Read the model definition and answer for the solid it produces. Units are mm, in the model's axes. A direction names the side the tool comes from. Coordinates: 2 decimals unless noted, no trailing zeros. Write each loop counter-clockwise with the first axis right and the second up, starting at its lowest first coordinate (ties: lowest second). Pieces come first, ordered by that corner, then holes.
(1) Which of the six approach directions +Z, -Z, +X, -X, +Y, -Y give full straight-line access (tool end or side, diameter ignored) to faces 4 (the flat face through (-0.58, 10, -10.35)), 5 (the flat face through (-0.55, 0, -10.35)), 6 (the flat face through (0, 5, -10.2))?
(2) The part is cut by section A-A, the plane x = -24.5. Determine the outline of the cut face in (y, z), and give its area (3 significant figures).
(3) The part is cut by section C-C, the plane z = -5. State how many separate pieces and enclosed holes the cut face has, and give its area (3 significant figures).
(4) The part is cut by section B-B, the plane y = 2.75. Determine the outline of the cut face in (x, z).
(5) Straight lines are drawn through the part: line 1 along X through (y, z) = (4, 5); line 2 along X through (y, z) = (-6.5, -9); line 3 along X through (y, z) = (2.5, 7). For each, find the intervals that lie inside material, in ascending order.
(6) Determine the mould class of faces 1 (the cylindrical face through (-43, -9, 5.8)), 2 (the cylindrical face through (-45.07, -2.68, -13.7)), 3 (the cylindrical face through (-45.07, 8.5, -0.21)) for opening direction Z: pulls with the +Z half, pulls with the -Z half, needs draft (parallel to the pull), parting line crosses it, or undercut.
(7) Given pin 1 (15 mm diameter, centred on x = -16, z = -4, fed in from -Y); pin 2 (1.5 mm diameter, centred on y = 7, z = 3.5, fed in from -X), each flat-ended and moving along its own axis, determine where each tip first touches the part or whether it passes through.
(8) The part is cut by section D-D, the plane y = -2.5. Determine the outline of the cut face in (x, z).
```python
from build123d import *

# Parameters (mm, degrees)
SKETCH_1_W          = 93
SKETCH_1_H          = 30.4
SKETCH_1_R          = 2.2
SKETCH_1_W_2        = 40.4
SKETCH_1_H_2        = 20.4
EXTRUDE_1_DEPTH     = 10
SKETCH_2_W          = 7
SKETCH_2_H          = 30.4
EXTRUDE_2_DEPTH     = 15
SKETCH_4_R          = 1.7
CUT_EXTRUDE_2_DEPTH = 96.420333263
FILLET_1_R          = 5


with BuildPart() as part:
    # 草图1 → 凸台-拉伸1 (new body)
    with BuildSketch(Plane(origin=(0, 0, 0), x_dir=(1, 0, 0), z_dir=(0, 1, 0))):
        Rectangle(SKETCH_1_W, SKETCH_1_H)
        with Locations(Location((-24.5, 5, 0), (0, 0, 270))):
            Circle(SKETCH_1_R, mode=Mode.SUBTRACT)
        with Locations(Location((-24.5, -5, 0), (0, 0, 270))):
            Circle(SKETCH_1_R, mode=Mode.SUBTRACT)
        with Locations(Location((24.5, -5, 0), (0, 0, 270))):
            Circle(SKETCH_1_R, mode=Mode.SUBTRACT)
        with Locations(Location((24.5, 5, 0), (0, 0, 270))):
            Circle(SKETCH_1_R, mode=Mode.SUBTRACT)
        Rectangle(SKETCH_1_W_2, SKETCH_1_H_2, mode=Mode.SUBTRACT)
    extrude(amount=EXTRUDE_1_DEPTH)

    # 草图2 → 凸台-拉伸2 (add)
    with BuildSketch(Plane.XZ):
        with Locations((-43, 0)):
            Rectangle(SKETCH_2_W, SKETCH_2_H)
        with Locations((43, 0)):
            Rectangle(SKETCH_2_W, SKETCH_2_H)
    extrude(amount=EXTRUDE_2_DEPTH)

    # 草图4 → 切除-拉伸2 (cut, through all)
    with BuildSketch(Plane.ZY.offset(46.5)):
        with Locations((-5, -7.5)):
            Circle(SKETCH_4_R)
        with Locations((5, -7.5)):
            Circle(SKETCH_4_R)
    extrude(amount=-CUT_EXTRUDE_2_DEPTH, mode=Mode.SUBTRACT)

    # 圆角1
    fillet_1_edges = [part.edges().sort_by_distance(p)[0] for p in [
        (46.5, 10, 0),
        (-46.5, 10, 0),
        (-46.5, -2.5, -15.2),
        (46.5, -2.5, -15.2),
        (46.5, -2.5, 15.2),
        (-46.5, -2.5, 15.2),
    ]]
    fillet(fillet_1_edges, radius=FILLET_1_R)


solid = part.part
```
Computed:
1. face 4: +Z, -Z, +X, -X, +Y
1. face 5: +Z, -Z, -Y
1. face 6: +Y, -Y
2. outline: (0, -15.2) - (10, -15.2) - (10, -7.2) - (0, -7.2) - close; (0, -2.8) - (10, -2.8) - (10, 2.8) - (0, 2.8) - close; (0, 7.2) - (10, 7.2) - (10, 15.2) - (0, 15.2) - close
2. area: 216 mm2
3. separate pieces: 6
3. enclosed holes: 0
3. area: 590 mm2
4. outline: (-46.5, -10.2) arc R5 ccw to (-41.5, -15.2) - (41.5, -15.2) arc R5 ccw to (46.5, -10.2) - (46.5, 10.2) arc R5 ccw to (41.5, 15.2) - (-41.5, 15.2) arc R5 ccw to (-46.5, 10.2) - close; hole circle Ø4.4 at (-24.5, -5); hole circle Ø4.4 at (-24.5, 5); hole (-20.2, -10.2) - (20.2, -10.2) - (20.2, 10.2) - (-20.2, 10.2) - close; hole circle Ø4.4 at (24.5, -5); hole circle Ø4.4 at (24.5, 5)
5. line 1: x = -46.5 to -26.7, -22.3 to -20.2, 20.2 to 22.3, 26.7 to 46.5
5. line 2: x = -46.5 to -39.5, 39.5 to 46.5
5. line 3: x = -46.5 to -25.42, -23.58 to -20.2, 20.2 to 23.58, 25.42 to 46.5
6. face 1: undercut
6. face 2: pulls with the -Z half
6. face 3: needs draft
7. pin 1: stops at y = 0
7. pin 2: stops at x = -46.34
8. outline: (-46.5, -10.2) arc R5 ccw to (-41.5, -15.2) - (-39.5, -15.2) - (-39.5, 15.2) - (-41.5, 15.2) arc R5 ccw to (-46.5, 10.2) - close; (39.5, -15.2) - (41.5, -15.2) arc R5 ccw to (46.5, -10.2) - (46.5, 10.2) arc R5 ccw to (41.5, 15.2) - (39.5, 15.2) - close
